Check sheet for the drawn part. Datum: minimum x, y, z corner. Units: mm. Round coordinates to 2 decimals unless told otherwise and drop trailing zeros. Order: outer loops, then holes, each group sorted by start corner. A loop starts at its lowest first (then second) coordinate and runs counter-clockwise, first axis right, second up.
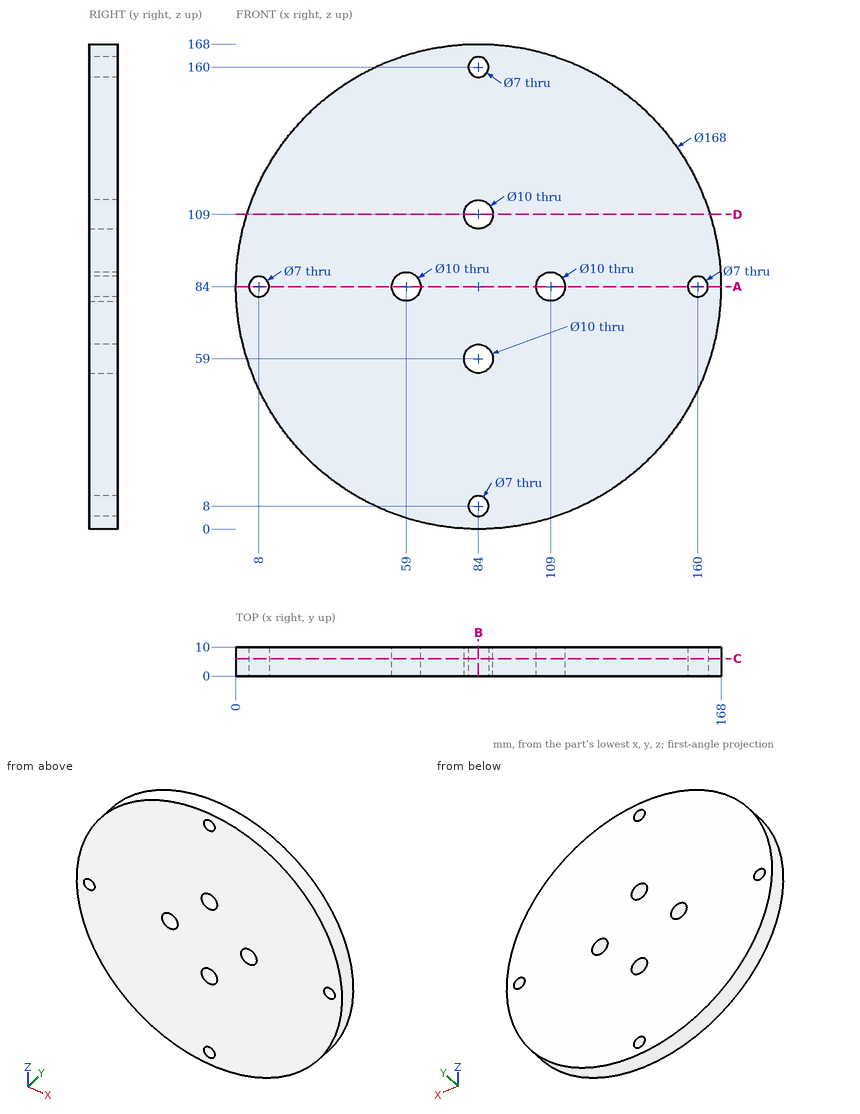
(1) Material ranges on line 1 (X direction, y = 6.75, z = 84); line 2 (Z direction, x = 107, y = 8); line 3 (X direction, y = 6.25, z = 160), recorded low to high.
Returned:
line 1: x = 0 to 4.5, 11.5 to 54, 64 to 104, 114 to 156.5, 163.5 to 168
line 2: z = 3.21 to 79.42, 88.58 to 164.79
line 3: x = 48.22 to 80.5, 87.5 to 119.78
(2) Sectioned sample at D-D, the plane z = 109. Record the cut outline in (x, y).
Returned:
outline: (3.81, 0) - (79, 0) - (79, 10) - (3.81, 10) - close; (89, 0) - (164.19, 0) - (164.19, 10) - (89, 10) - close
(3) Sectioned sample at A-A, the plane z = 84. Record the cut outline in (x, y).
Returned:
outline: (0, 0) - (4.5, 0) - (4.5, 10) - (0, 10) - close; (11.5, 0) - (54, 0) - (54, 10) - (11.5, 10) - close; (64, 0) - (104, 0) - (104, 10) - (64, 10) - close; (114, 0) - (156.5, 0) - (156.5, 10) - (114, 10) - close; (163.5, 0) - (168, 0) - (168, 10) - (163.5, 10) - close
(4) Sectioned sample at C-C, the plane y = 6. Give the number of separate pieces and of enclosed holes in the cut face, and give its area (3 significant figures).
Returned:
separate pieces: 1
enclosed holes: 8
area: 21,700 mm2
(5) Sectioned sample at B-B, the plane x = 84. Record the cut outline in (y, z), and give its area (3 significant figures).
Returned:
outline: (0, 0) - (10, 0) - (10, 4.5) - (0, 4.5) - close; (0, 11.5) - (10, 11.5) - (10, 54) - (0, 54) - close; (0, 64) - (10, 64) - (10, 104) - (0, 104) - close; (0, 114) - (10, 114) - (10, 156.5) - (0, 156.5) - close; (0, 163.5) - (10, 163.5) - (10, 168) - (0, 168) - close
area: 1,340 mm2
(6) Depth check by flat-ended pin: P1, Ø1, axis at y = 5.5, z = 100.5, coming from the -X side; P2, Ø6.5, axis at x = 84, z = 160, coming from the +Y side; P3, Ø1.5, axis at x = 37, y = 3, coming from the -Z side; P4, Ø6, axis at y = 7, z = 94.5, coming from the -X side. Enter the tip coordinate at first touch or a pass-through.
Returned:
P1: stops at x = 1.54
P2: passes through
P3: stops at z = 13.88
P4: stops at x = 0.34
